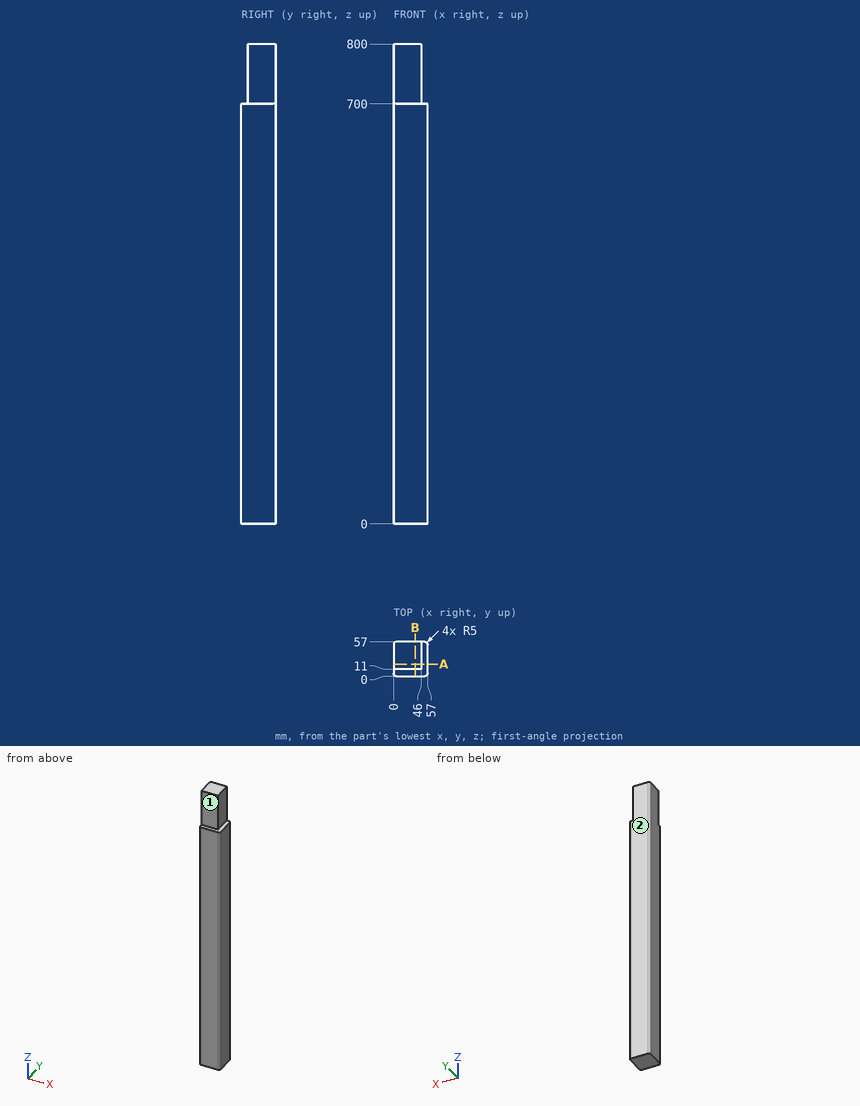
Verification items for this drawing (mm, ordinates from the low corner). A direction names the side the tool comes from. Coordinates: 2 decimals unless noted, no trailing zeros. Loops run counter-clockwise (first coordinate to the right, second up) from the corner with the lowest first, then second, coordinate; pieces in that order, holes last. Notation, with made-up numbers: (40.25, -38.5) -> (68.25, -38.5) arc R13 cw to (68.25, -15.5) -> close; hole circle Ø1 at (1.5, 23). An arc over 180 degrees is marked (long way). Answer in a Markdown table with one row per item. Add a question column.
1. Access from +Z, -Z, +X, -X, +Y, -Y to the whole of each face (thin tool, end or side, straight path). Record for the marked faces 1 and 2.
2. Section check B-B, the plane x = 36. Enter the section's corners in (y, z).
3. Depth check by flat-ended pin: P1, Ø14, axis at y = 40.5, z = 771, coming from the +X side. Enter the tip coordinate at first touch or a pass-through.
4. Section check A-A, the plane y = 20. Enter the section's corners in (x, z), then the cut area to 3 significant figures.
5. Material ranges on probe 1 along X at (y, z) = (4.5, 231); probe 2 along Z at (x, y) = (4.5, 7); probe 3 along X at (y, z) = (32, 744), recorded low to high. Write a range as [from, to].
Derived:
| question | item | result |
|---|---|---|
| 1 | face 1 | +Z, +X, -X, -Y |
| 1 | face 2 | +Z, -Z, +X, -X, +Y |
| 2 | outline | (0, 0) -> (57, 0) -> (57, 800) -> (11, 800) -> (11, 700) -> (0, 700) -> close |
| 3 | P1 | stops at x = 46 |
| 4 | outline | (0, 0) -> (57, 0) -> (57, 700) -> (46, 700) -> (46, 800) -> (0, 800) -> close |
| 4 | area | 44,500 mm² |
| 5 | probe 1 | x = [0.03, 56.97] |
| 5 | probe 2 | z = [0, 700] |
| 5 | probe 3 | x = [0, 46] |
